Work out the finished part from the listing and answer in its coordinate system (mm). A direction names the side the tool comes from. Coordinates: 2 decimals unless noted, no trailing zeros. Loops run counter-clockwise (first coordinate to the right, second up) from the corner with the lowest first, then second, coordinate; pieces in that order, holes last. Notation, with made-up numbers: (-28, -36.5) -> (-1, -36.5) arc R15 cw to (-1, -18.5) -> close; hole circle Ø4 at (-15.5, -18). An arc over 180 degrees is marked (long way). Use a Markdown table: item, result.
from build123d import *

# Parameters (mm, degrees)
BOSS_EXTRUDE1_DEPTH = 6
SKETCH2_W           = 66
SKETCH2_H           = 66
SKETCH2_R           = 1.705
SKETCH2_W_2         = 50
SKETCH2_H_2         = 50
BOSS_EXTRUDE2_DEPTH = 60
SKETCH4_W           = 7
SKETCH4_H           = 7
CUT_EXTRUDE2_DEPTH  = 52
SKETCH5_W           = 33
SKETCH5_H           = 8
SKETCH5_W_2         = 8
SKETCH5_H_2         = 33
CUT_EXTRUDE3_DEPTH  = 45


with BuildPart() as part:
    # Sketch1 → Boss-Extrude1 (new body)
    with BuildSketch(Plane(origin=(0, 0, 0), x_dir=(1, 0, 0), z_dir=(0, 1, 0))):
        Polygon((-20, 80), (20, 80), (20, 35), (35, 35), (35, 20), (80, 20), (80, -20), (35, -20), (35, -35), (20, -35), (20, -80), (-20, -80), (-20, -35), (-35, -35), (-35, -20), (-80, -20), (-80, 20), (-35, 20), (-35, 35), (-20, 35), align=None)
    extrude(amount=-BOSS_EXTRUDE1_DEPTH)

    # Sketch2 → Boss-Extrude2 (add)
    with BuildSketch(Plane(origin=(0, 0, 0), x_dir=(1, 0, 0), z_dir=(0, 1, 0))):
        Rectangle(SKETCH2_W, SKETCH2_H)
        with Locations(Location((29, 29, 0), (0, 0, 270))):
            Circle(SKETCH2_R, mode=Mode.SUBTRACT)
        with Locations(Location((-29, 29, 0), (0, 0, 270))):
            Circle(SKETCH2_R, mode=Mode.SUBTRACT)
        with Locations(Location((29, -29, 0), (0, 0, 270))):
            Circle(SKETCH2_R, mode=Mode.SUBTRACT)
        with Locations(Location((-29, -29, 0), (0, 0, 270))):
            Circle(SKETCH2_R, mode=Mode.SUBTRACT)
        Rectangle(SKETCH2_W_2, SKETCH2_H_2, mode=Mode.SUBTRACT)
    extrude(amount=BOSS_EXTRUDE2_DEPTH)

    # Sketch4 → Cut-Extrude2 (cut)
    with BuildSketch(Plane(origin=(0, 0, 0), x_dir=(1, 0, 0), z_dir=(0, 1, 0))):
        with Locations((-29.5, 29.5)):
            Rectangle(SKETCH4_W, SKETCH4_H)
        with Locations((29.5, 29.5)):
            Rectangle(SKETCH4_W, SKETCH4_H)
        with Locations((29.5, -29.5)):
            Rectangle(SKETCH4_W, SKETCH4_H)
        with Locations((-29.5, -29.5)):
            Rectangle(SKETCH4_W, SKETCH4_H)
    extrude(amount=CUT_EXTRUDE2_DEPTH, mode=Mode.SUBTRACT)

    # Sketch5 → Cut-Extrude3 (cut)
    with BuildSketch(Plane(origin=(0, 0, 0), x_dir=(1, 0, 0), z_dir=(0, 1, 0))):
        with Locations((0, 29)):
            Rectangle(SKETCH5_W, SKETCH5_H)
        with Locations((0, -29)):
            Rectangle(SKETCH5_W, SKETCH5_H)
        with Locations((29, 0)):
            Rectangle(SKETCH5_W_2, SKETCH5_H_2)
        with Locations((-29, 0)):
            Rectangle(SKETCH5_W_2, SKETCH5_H_2)
    extrude(amount=CUT_EXTRUDE3_DEPTH, mode=Mode.SUBTRACT)


solid = part.part
Q1. For faces 4 (the flat face through (-30.33, 52, -30.33)), 5 (the flat face through (-16.5, 22, 29)), 6 (the flat face through (-29, 45, 0)), 7 (the flat face through (29, 26, -26)), determine the directions among +Z, -Z, +X, -X, +Y, -Y from which every point of the face is accessible in a straight line to the end or side of a thin tool.
Solved:
| item | result |
|---|---|
| face 4 | -Z, -X |
| face 5 | +Z, -Z |
| face 6 | +X, -X |
| face 7 | -Z, +X |
Q2. Section A-A on x = 12 is taken. Determine the outline of the cut face in (y, z), and give its area (3 significant figures).
Solved:
| item | result |
|---|---|
| outline | (-6, -80) -> (0, -80) -> (0, 80) -> (-6, 80) -> close; (45, -33) -> (60, -33) -> (60, -25) -> (45, -25) -> close; (45, 25) -> (60, 25) -> (60, 33) -> (45, 33) -> close |
| area | 1,200 mm² |
Q3. Section B-B on y = 47 is taken. Determine the outline of the cut face in (x, z), and give its area (3 significant figures).
Solved:
| item | result |
|---|---|
| outline | (-33, -26) -> (-26, -26) -> (-26, -33) -> (26, -33) -> (26, -26) -> (33, -26) -> (33, 26) -> (26, 26) -> (26, 33) -> (-26, 33) -> (-26, 26) -> (-33, 26) -> close; hole (-25, -25) -> (25, -25) -> (25, 25) -> (-25, 25) -> close |
| area | 1,660 mm² |
Q4. Determine the mould class of faces 1 (the flat face through (-6, 50, 25)), 2 (the flat face through (29, 22, 16.5)), 3 (the flat face through (26, 26, 30)) for opening direction X: pulls with the +X half, pulls with the -X half, needs draft (parallel to the pull), parting line crosses it, or undercut.
Solved:
| item | result |
|---|---|
| face 1 | undercut |
| face 2 | needs draft |
| face 3 | pulls with the +X half |
Q5. Consider line 1 (X direction, y = 56.5, z = -29) (3 decimals); line 2 (Z direction, x = -6, y = 51). Determine where each line is inside the solid, lowest interval first. Write a range as [from, to].
Solved:
| item | result |
|---|---|
| line 1 | [-33, -30.705], [-27.295, 27.295], [30.705, 33] |
| line 2 | [-33, -25], [25, 33] |
Q6. Section C-C on z = 11 is taken. Determine the outline of the cut face in (x, y).
Solved:
| item | result |
|---|---|
| outline | (-80, -6) -> (80, -6) -> (80, 0) -> (-80, 0) -> close; (-33, 45) -> (-25, 45) -> (-25, 60) -> (-33, 60) -> close; (25, 45) -> (33, 45) -> (33, 60) -> (25, 60) -> close |
Q7. Given pin 1 Ø10 at (y, z) = (27.5, 32.5) entering from -X; pin 2 Ø5 at (x, y) = (49.5, -3) entering from +Z; pin 3 Ø2.5 at (x, y) = (31, 30.5) entering from +Z; pin 4 Ø6 at (x, y) = (1, 3.5) entering from -Z, each flat-ended and moving along its own axis, determine where each tip first touches the part or whether it passes through.
Solved:
| item | result |
|---|---|
| pin 1 | x = -26 |
| pin 2 | z = 20 |
| pin 3 | z = 26 |
| pin 4 | through |
Q8. Section D-D on y = 25.5 is taken. State how many separate pieces and enclosed holes the cut face has, and give its area (3 significant figures).
Solved:
| item | result |
|---|---|
| separate pieces | 4 |
| enclosed holes | 0 |
| area | 604 mm² |
